Could you check a few things on this drawing? It's one solid part, dimensions in mm from its lowest x, y, z. Round coordinates to 2 decimals unless told otherwise and drop trailing zeros. Write each loop counter-clockwise with the first axis right and the second up, starting at its lowest first coordinate (ties: lowest second). Pieces come first, ordered by that corner, then holes. Notation, with made-up numbers: (46, 19) - (97, 19) arc R18 ccw to (97, 30) - close; hole circle Ø1 at (-23, 15). An arc over 180 degrees is marked (long way). Use one line per item in the form item = value. Start each with the question number.
1. I want a section at B-B, the plane x = 15.5. List the corners of the cut face in (y, z) for me (1 decimal).
2. I want a section at A-A, the plane y = 14.25. List the corners of the cut face in (x, z) for me.
3. If I drill on line 1 along Y through (x, z) = (15, 2) (1 decimal); line 2 along X through (y, z) = (19, 0.75) (1 decimal); line 3 along Y through (x, z) = (14, 4.25), over which ranges is the centre line in solid material (lowest first)?
4. We'd pull the mould along X, two halves only. Please class the marked faces 1, 2 and 3: +X half, -X half, draft (parallel to the pull), parting line (faces both ways), or undercut.
5. I want a section at D-D, the plane x = 22. List the corners of the cut face in (y, z) for me.
6. Will these pins go through, and if not, where does the flat tip stop? pin 1 (3 mm diameter, centred on x = 15.5, y = 15.5, fed in from -Z); pin 2 (1.5 mm diameter, centred on y = 19.5, z = 2.5, fed in from -X).
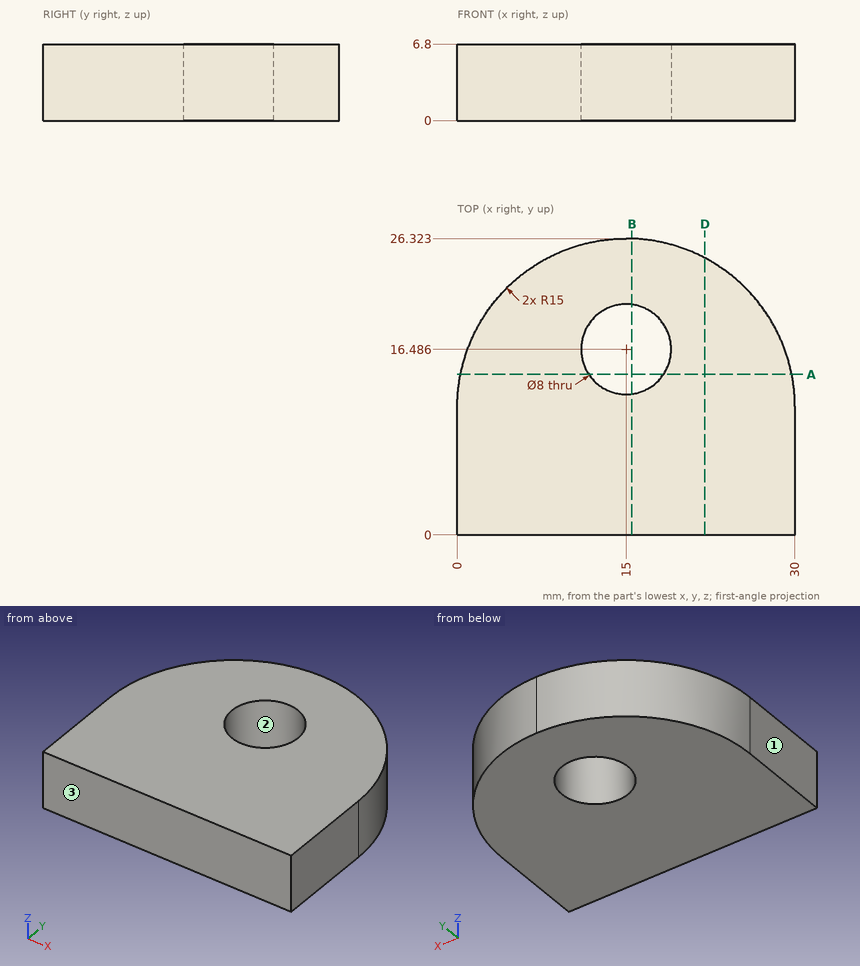
Model answer:
q1.outline = (0, 0) - (12.5, 0) - (12.5, 6.8) - (0, 6.8) - close; (20.5, 0) - (26.3, 0) - (26.3, 6.8) - (20.5, 6.8) - close
q2.outline = (0.29, 0) - (11.68, 0) - (11.68, 6.8) - (0.29, 6.8) - close; (18.32, 0) - (29.71, 0) - (29.71, 6.8) - (18.32, 6.8) - close
q3.line_1 = 0 to 12.5, 20.5 to 26.3
q3.line_2 = 2.1 to 11.9, 18.1 to 27.9
q3.line_3 = 0 to 12.61, 20.36 to 26.29
q4.face_1 = -X half
q4.face_2 = undercut
q4.face_3 = draft
q5.outline = (0, 0) - (24.59, 0) - (24.59, 6.8) - (0, 6.8) - close
q6.pin_1 = through
q6.pin_2 = 1.97
